```python
from build123d import *

# Parameters (mm, degrees)
F0_R     = 71.187924
F0_R_2   = 65.063911
F1_DEPTH = 718.82
F2_R     = 39.27729
F2_R_2   = 26.178049
F3_DEPTH = 157.48


with BuildPart() as f1:
    # F0 (on Front) → F1 (new body)
    with BuildSketch(Plane.XZ):
        Circle(F0_R)
        Circle(F0_R_2, mode=Mode.SUBTRACT)
    extrude(amount=F1_DEPTH)

    # F2 (on Right) → F3 (join)
    with BuildSketch(Plane.YZ):
        Circle(F2_R)
        Circle(F2_R_2, mode=Mode.SUBTRACT)
        Circle(F2_R_2)
    extrude(amount=F3_DEPTH)


solid = f1.part
```
Check sheet for the modelled part. Datum: model origin and axes. Units: mm. A direction names the side the tool comes from. Give positions to 0.01 mm unless a question says otherwise; leave off trailing zeros. Order: outer loops, then holes, each group sorted by start corner. A loop starts at its lowest first (then second) coordinate and runs counter-clockwise, first axis right, second up. Notation, with made-up numbers: M 19.25,51.25 L 39.25,51.25 A17 cw 39.25,78.25 Z; hole C 65.25,27 d1. An arc over 180 degrees is marked long. Answer in a Markdown table with one row per item. Add a question column.
Q1. Sectioned sample at B-B, the plane x = 24.5. Record the boundary of the cut face in (y, z), and give its area (3 significant figures).
Q2. Sectioned sample at D-D, the plane z = 30.5. Record the boundary of the cut face in (x, y).
Q3. Sectioned sample at A-A, the plane z = 0. Record the boundary of the cut face in (x, y), and give its area (3 significant figures).
Q4. Sectioned sample at C-C, the plane y = -191. Record the boundary of the cut face in (x, z), and give its area (3 significant figures).
Q5. Access from +Z, -Z, +X, -X, +Y, -Y to the whole of each face (thin tool, end or side, straight path). Record for faces 1 (the cylindrical face through (-8.47, -354.38, 64.51)), 2 (the flat face through (157.48, -1, 1)).
Q6. Thickness scan on L1, parallel to Z at x = 0, y = -546; L2, parallel to Z at x = 3, y = -56.5. Record the ranges inside material, lowest first.
Q7. Gauge pin test, flat ends, axial feed: pin 1 Ø6 at (x, z) = (92.5, -30.5) entering from -Y; pin 2 Ø1 at (x, z) = (74, 25.5) entering from -Y; pin 3 Ø4 at (x, y) = (10.5, -510.5) entering from +Z. Record the tip position at first contact, or that the pin passes through.
Q8. Release check for a two-part mould opening along Z. For faces 3 (the cylindrical face through (-9.27, -354.38, 70.58)), 4 (the cylindrical face through (77.64, 18.12, -34.85)), 5 (the flat face through (-64, 0, 16)), 6 (the flat face through (0, -1, 1)) record: released by +Z, released by -Z, zero draft, split by the parting line, or undercut.
Verdict:
| question | item | result |
|---|---|---|
| 1 | outline | M -718.82,-66.84 L 0,-66.84 L 0,-60.27 L -718.82,-60.27 Z; M -718.82,60.27 L 0,60.27 L 0,66.84 L -718.82,66.84 Z; C 0,0 d78.55 |
| 1 | area | 14,300 mm² |
| 2 | outline | M -64.32,-718.82 L -57.47,-718.82 L -57.47,0 L -64.32,0 Z; M 0,-24.75 L 57.47,-24.75 L 57.47,-718.82 L 64.32,-718.82 L 64.32,-24.75 L 157.48,-24.75 L 157.48,24.75 L 0,24.75 Z |
| 3 | outline | M -71.19,-718.82 L -65.06,-718.82 L -65.06,0 L -71.19,0 Z; M 0,-39.28 L 65.06,-39.28 L 65.06,-718.82 L 71.19,-718.82 L 71.19,-39.28 L 157.48,-39.28 L 157.48,39.28 L 0,39.28 Z |
| 3 | area | 20,900 mm² |
| 4 | outline | C 0,0 d142.38; hole C 0,0 d130.13 |
| 4 | area | 2,620 mm² |
| 5 | face 1 | -Y |
| 5 | face 2 | +Z, -Z, +X, +Y, -Y |
| 6 | L1 | -71.19 to -65.06, 65.06 to 71.19 |
| 6 | L2 | -71.12 to -64.99, 64.99 to 71.12 |
| 7 | pin 1 | y = -28.04 |
| 7 | pin 2 | y = -30.29 |
| 7 | pin 3 | z = 70.68 |
| 8 | face 3 | split by the parting line |
| 8 | face 4 | undercut |
| 8 | face 5 | zero draft |
| 8 | face 6 | undercut |
